Input: part model. Units: mm. Frame: model coordinates. A direction names the side the tool comes from. Coordinates: 2 decimals unless noted, no trailing zeros. Loops run counter-clockwise (first coordinate to the right, second up) from the corner with the lowest first, then second, coordinate; pieces in that order, holes last. Notation, with made-up numbers: (-34, 89) - (-11, 89) arc R13 ccw to (-11, 108) - close; hole circle Ø7 at (66, -31.5). An arc over 180 degrees is marked (long way). Use one line per item in the form item = value.
from build123d import *

# Parameters (mm, degrees)
SKETCH_1_W          = 15
SKETCH_1_H          = 15
SKETCH_1_W_2        = 12
SKETCH_1_H_2        = 12
EXTRUDE_1_DEPTH     = 600
SKETCH_3_R          = 2
CUT_EXTRUDE_2_DEPTH = 25
SKETCH_4_R          = 2.75
CUT_EXTRUDE_3_DEPTH = 20
SKETCH_6_R          = 2
CUT_EXTRUDE_4_DEPTH = 20
SKETCH_9_R          = 5
CUT_EXTRUDE_7_DEPTH = 10


with BuildPart() as part:
    # ｽｹｯﾁ1 → ﾎﾞｽ - 押し出し1 (new body)
    with BuildSketch(Plane.XY):
        Rectangle(SKETCH_1_W, SKETCH_1_H)
        Rectangle(SKETCH_1_W_2, SKETCH_1_H_2, mode=Mode.SUBTRACT)
    extrude(amount=EXTRUDE_1_DEPTH)

    # ｽｹｯﾁ3 → ｶｯﾄ - 押し出し2 (cut)
    with BuildSketch(Plane(origin=(0, 7.5, 0), x_dir=(1, 0, 0), z_dir=(0, 1, 0))):
        with Locations((0, -7.5)):
            Circle(SKETCH_3_R)
        with Locations((0, -592.5)):
            Circle(SKETCH_3_R)
    extrude(amount=-CUT_EXTRUDE_2_DEPTH, mode=Mode.SUBTRACT)

    # ｽｹｯﾁ4 → ｶｯﾄ - 押し出し3 (cut)
    with BuildSketch(Plane(origin=(7.5, 0, 0), x_dir=(0, 0, -1), z_dir=(1, 0, 0))):
        with Locations((-536, 0)):
            Circle(SKETCH_4_R)
        with Locations((-501, 0)):
            Circle(SKETCH_4_R)
        with Locations((-99, 0)):
            Circle(SKETCH_4_R)
        with Locations((-64, 0)):
            Circle(SKETCH_4_R)
    extrude(amount=-CUT_EXTRUDE_3_DEPTH, mode=Mode.SUBTRACT)

    # ｽｹｯﾁ6 → ｶｯﾄ - 押し出し4 (cut)
    with BuildSketch(Plane(origin=(0, 7.5, 0), x_dir=(1, 0, 0), z_dir=(0, 1, 0))):
        with Locations((0, -336.5)):
            Circle(SKETCH_6_R)
        with Locations((0, -263.5)):
            Circle(SKETCH_6_R)
    extrude(amount=-CUT_EXTRUDE_4_DEPTH, mode=Mode.SUBTRACT)

    # ｽｹｯﾁ9 → ｶｯﾄ - 押し出し7 (cut)
    with BuildSketch(Plane.XZ.offset(7.5)):
        with Locations((0, 592.5)):
            Circle(SKETCH_9_R)
        with Locations((0, 336.5)):
            Circle(SKETCH_9_R)
        with Locations((0, 263.5)):
            Circle(SKETCH_9_R)
        with Locations((0, 7.5)):
            Circle(SKETCH_9_R)
    extrude(amount=-CUT_EXTRUDE_7_DEPTH, mode=Mode.SUBTRACT)


solid = part.part
Q1. First-contact query: P1, Ø6, axis at x = 0, z = 592.5, coming from the -Y side. Flat tip, straight axial feed; report the tip coordinate or a pass-through.
Check values:
P1 = 6
Q2. Cut plane A-A, the plane z = 367. Return loops of the section in (x, y), then the cut area to 3 significant figures.
Check values:
outline = (-7.5, -7.5) - (7.5, -7.5) - (7.5, 7.5) - (-7.5, 7.5) - close; hole (-6, -6) - (6, -6) - (6, 6) - (-6, 6) - close
area = 81.0 mm²
Q3. Ray query, line 1 along Z through (x, y) = (0, 7.2); line 2 along Z through (x, y) = (0, -6.4); line 3 along Y through (x, z) = (3, 169). Return the intervals inside material, ascending. Write a range as [from, to].
Check values:
line_1 = [0, 5.5], [9.5, 261.5], [265.5, 334.5], [338.5, 590.5], [594.5, 600]
line_2 = [0, 2.5], [12.5, 258.5], [268.5, 331.5], [341.5, 587.5], [597.5, 600]
line_3 = [-7.5, -6], [6, 7.5]
Q4. Pull-direction query (Z, two-part tool) for faces 1 (the cylindrical face through (-0.651, -6.76, 341.457)), 2 (the flat face through (0, -7.5, 296)), 3 (the flat face through (-7, 0, 0)); classes: pulls with the +Z half, pulls with the -Z half, needs draft (parallel to the pull), parting line crosses it, or undercut.
Check values:
face_1 = undercut
face_2 = needs draft
face_3 = pulls with the -Z half
Q5. Set-up query: faces 4 (the flat face through (6, 0, 296)), 5 (the flat face through (0, 7.5, 296)), 6 (the cylindrical face through (-0.651, -6.76, 268.457)). Return all of +Z, -Z, +X, -X, +Y, -Y with unobstructed straight access to the full face (end or side cutting, diameter ignored); none if empty.
Check values:
face_4 = +Z, -Z
face_5 = +Z, -Z, +X, -X, +Y
face_6 = -Y
Q6. Cut plane B-B, the plane y = 0. Give the number of separate pieces and of enclosed holes in the cut face, then the cut area to 3 significant figures.
Check values:
separate_pieces = 10
enclosed_holes = 0
area = 1,730 mm²
